Geometry check sheet. Reference: the model listing, model coordinates, mm. Coordinates: 2 decimals unless noted, no trailing zeros. Order: outer loops, then holes, each group sorted by start corner. A loop starts at its lowest first (then second) coordinate and runs counter-clockwise, first axis right, second up. Notation, with made-up numbers: M 87.25,-23.75 L 106.25,-23.75 A28 ccw 106.25,12.25 Z; hole C 4,27.25 d2. An arc over 180 degrees is marked long. Use CSV: the item, a comma, the result in double quotes. Start each with the question number.
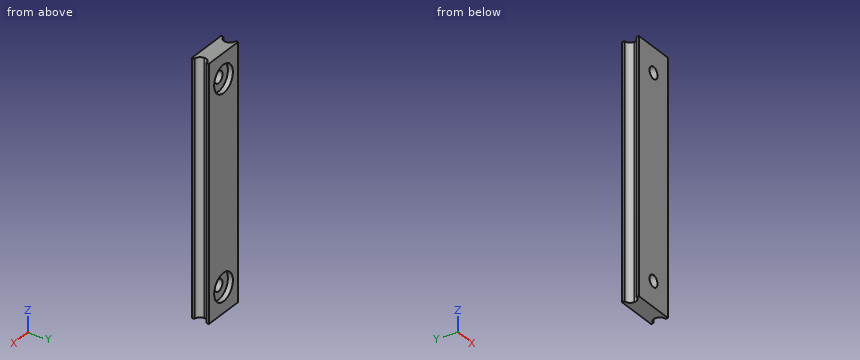
```python
from build123d import *

# Parameters (mm, degrees)
BOSS_EXTRUDE1_DEPTH = 25
SKETCH2_R           = 1.175
CUT_EXTRUDE1_DEPTH  = 4.41
SKETCH3_R           = 2.75
CUT_EXTRUDE2_DEPTH  = 1


with BuildPart() as part:
    # Sketch1 → Boss-Extrude1 (new body, symmetric)
    with BuildSketch(Plane.XY):
        with BuildLine():
            Line((-3.14, 0.055), (-3.14, -0.055))
            ThreePointArc((-3.14, -0.055), (-3.476827202, -0.868172798), (-4.29, -1.205))
            Line((-4.29, -1.205), (-4.29, -1.705))
            Line((-4.29, -1.705), (4.29, -1.705))
            Line((4.29, -1.705), (4.29, -1.205))
            ThreePointArc((4.29, -1.205), (3.476827202, -0.868172798), (3.14, -0.055))
            Line((3.14, -0.055), (3.14, 0.055))
            ThreePointArc((3.14, 0.055), (3.476827202, 0.868172798), (4.29, 1.205))
            Line((4.29, 1.205), (4.29, 1.705))
            Line((4.29, 1.705), (-4.29, 1.705))
            Line((-4.29, 1.705), (-4.29, 1.205))
            ThreePointArc((-4.29, 1.205), (-3.476827202, 0.868172798), (-3.14, 0.055))
        make_face()
    extrude(amount=BOSS_EXTRUDE1_DEPTH, both=True)

    # Sketch2 → Cut-Extrude1 (cut, through all)
    with BuildSketch(Plane(origin=(0, 1.705, 0), x_dir=(1, 0, 0), z_dir=(0, 1, 0))):
        with Locations((0, 20)):
            Circle(SKETCH2_R)
    cut_extrude1 = extrude(amount=-CUT_EXTRUDE1_DEPTH, mode=Mode.SUBTRACT)

    # Sketch3 → Cut-Extrude2 (cut)
    with BuildSketch(Plane(origin=(0, 1.705, 0), x_dir=(1, 0, 0), z_dir=(0, 1, 0))):
        with Locations((0, 20)):
            Circle(SKETCH3_R)
    cut_extrude2 = extrude(amount=-CUT_EXTRUDE2_DEPTH, mode=Mode.SUBTRACT)

    # Mirror1: Cut-Extrude1, Cut-Extrude2 across plane
    add(cut_extrude1.mirror(Plane.XY), mode=Mode.SUBTRACT)
    add(cut_extrude2.mirror(Plane.XY), mode=Mode.SUBTRACT)


solid = part.part
```
1) Gauge pin test, flat ends, axial feed: P1, Ø3, axis at x = 0.5, z = 21, coming from the +Y side (3 decimals); P2, Ø3, axis at x = 0, z = 20, coming from the -Y side (3 decimals). Record the tip position at first contact, or that the pin passes through.
2) Material ranges on line 1 along Z through (x, y) = (0, -0.8) (3 decimals); line 2 along Z through (x, y) = (0, 1.35); line 3 along X through (y, z) = (0.15, -20) (3 decimals), recorded low to high.
3) Section check C-C on y = -0.6. Record the boundary of the cut face in (x, z) (3 decimals), then the cut area to 3 significant figures.
4) Section check D-D on z = 6. Record the boundary of the cut face in (x, y) (3 decimals).
5) Section check A-A on x = 0. Record the boundary of the cut face in (y, z) (3 decimals).
6) Section check B-B on z = 20. Record the boundary of the cut face in (x, y) (3 decimals), then the cut area to 3 significant figures.
Results are:
1,P1,"stops at y = 0.705"
1,P2,"stops at y = -1.705"
2,line 1,"z = -25 to -21.175, -18.825 to 18.825, 21.175 to 25"
2,line 2,"z = -25 to -22.75, -17.25 to 17.25, 22.75 to 25"
2,line 3,"x = -3.144 to -1.175, 1.175 to 3.144"
3,outline,"M -3.277,-25 L 3.277,-25 L 3.277,25 L -3.277,25 Z; hole C 0,-20 d2.35; hole C 0,20 d2.35"
3,area,"319 mm²"
4,outline,"M -4.29,-1.705 L 4.29,-1.705 L 4.29,-1.205 A1.15 cw 3.14,-0.055 L 3.14,0.055 A1.15 cw 4.29,1.205 L 4.29,1.705 L -4.29,1.705 L -4.29,1.205 A1.15 cw -3.14,0.055 L -3.14,-0.055 A1.15 cw -4.29,-1.205 Z"
5,outline,"M -1.705,-25 L 1.705,-25 L 1.705,-22.75 L 0.705,-22.75 L 0.705,-21.175 L -1.705,-21.175 Z; M -1.705,-18.825 L 0.705,-18.825 L 0.705,-17.25 L 1.705,-17.25 L 1.705,17.25 L 0.705,17.25 L 0.705,18.825 L -1.705,18.825 Z; M -1.705,21.175 L 0.705,21.175 L 0.705,22.75 L 1.705,22.75 L 1.705,25 L -1.705,25 Z"
6,outline,"M -4.29,-1.705 L -1.175,-1.705 L -1.175,0.705 L -2.75,0.705 L -2.75,1.705 L -4.29,1.705 L -4.29,1.205 A1.15 cw -3.14,0.055 L -3.14,-0.055 A1.15 cw -4.29,-1.205 Z; M 1.175,-1.705 L 4.29,-1.705 L 4.29,-1.205 A1.15 cw 3.14,-0.055 L 3.14,0.055 A1.15 cw 4.29,1.205 L 4.29,1.705 L 2.75,1.705 L 2.75,0.705 L 1.175,0.705 Z"
6,area,"13.7 mm²"
